Build history of the part. All positions in model axes, mm. A direction names the side the tool comes from. Round coordinates to 2 decimals unless told otherwise and drop trailing zeros. Write each loop counter-clockwise with the first axis right and the second up, starting at its lowest first coordinate (ties: lowest second). Pieces come first, ordered by that corner, then holes. Notation, with made-up numbers: (8.25, 21) - (32.25, 21) arc R25 ccw to (32.25, 49) - close; hole circle Ø8 at (72, 48). An arc over 180 degrees is marked (long way). Answer as a JSON object with one key per item and string values. Group by question number.
Item 1: Slice it at A-A, the plane x = 0. List the corners of the cut face in (y, z), then the cut area to 3 significant figures.
Item 2: Slice it at D-D, the plane y = -2.5. List the corners of the cut face in (x, z), then the cut area to 3 significant figures.
Item 3: Slice it at B-B, the plane y = 0. List the corners of the cut face in (x, z), then the cut area to 3 significant figures.
Item 4: Two-plate mould, pull along X, no slides. Class faces 6 (the flat face through (0, 2.524, 8)), 7 (the flat face through (-0.9, 2, -6)), 8 (the flat face through (0.9, 2, -6)): +X half, -X half, draft (parallel to the pull), parting line (faces both ways), or undercut.
Item 5: Probe line 1 (Y direction, x = 0, z = 5.75); line 2 (Z direction, x = -2.25, y = -0.5); line 3 (Z direction, x = -5.25, y = -5.5). List the from-to ranges inside material, lowest first. Write a range as from..to.
Item 6: Which spindle directions (+Z, -Z, +X, -X, +Y, -Y) get a long thin tool onto all of the face, cutting with end or side? Do faces 1 (the flat face through (-2, 0.9, -6)), 2 (the flat face through (0, 2.2, -6)), 3 (the flat face through (-0.9, -2, -6)), 4 (the flat face through (0, 0, 2)), 5 (the flat face through (0.9, -2, -6)). Say none if no direction does.
Item 7: Flat gauge pins, fed straight in: pin 1 (0.7 mm diameter, centred on y = -1.5, z = -4, fed in from -X); pin 2 (1 mm diameter, centred on x = -2, z = -6.5, fed in from +Y); pin 3 (6 mm diameter, centred on x = 3.5, z = 5, fed in from -Y). Where does each tip first touch, or does it go through?
Item 8: Slice it at C-C, the plane z = 5. List the corners of the cut face in (x, y), then the cut area to 3 significant figures.
from build123d import *

# Parameters (mm, degrees)
SKETCH_R     = 8
PAD_DEPTH    = 14
POCKET_DEPTH = 12
PAD001_DEPTH = 12


with BuildPart() as part:
    # Sketch → Pad (new body)
    with BuildSketch(Plane.XY):
        Circle(SKETCH_R)
    extrude(amount=PAD_DEPTH)

    # Sketch001 → Pocket (cut)
    with BuildSketch(Plane.XY.offset(14)):
        with BuildLine():
            Line((-1.8, 2.523886), (1.8, 2.523886))
            ThreePointArc((-1.8, 2.523886), (0, -3.1), (1.8, 2.523886))
        make_face()
    extrude(amount=-POCKET_DEPTH, mode=Mode.SUBTRACT)

    # Sketch002 → Pad001 (new body)
    with BuildSketch(Plane(origin=(0, 0, 0), x_dir=(1, 0, 0), z_dir=(0, 0, -1))):
        Polygon((-0.9, 2.2), (0.9, 2.2), (0.9, 0.9), (2.2, 0.9), (2.2, -0.9), (0.9, -0.9), (0.9, -2.2), (-0.9, -2.2), (-0.9, -0.9), (-2.2, -0.9), (-2.2, 0.9), (-0.9, 0.9), align=None)
    extrude(amount=PAD001_DEPTH)


solid = part.part
Geometry says:
{
 "1": {"outline": "(-8, 0) - (-2.2, 0) - (-2.2, -12) - (2.2, -12) - (2.2, 0) - (8, 0) - (8, 14) - (2.52, 14) - (2.52, 2) - (-3.1, 2) - (-3.1, 14) - (-8, 14) - close", "area": "209 mm^2"},
 "2": {"outline": "(-7.6, 0) - (7.6, 0) - (7.6, 14) - (1.83, 14) - (1.83, 2) - (-1.83, 2) - (-1.83, 14) - (-7.6, 14) - close", "area": "169 mm^2"},
 "3": {"outline": "(-8, 0) - (-2.2, 0) - (-2.2, -12) - (2.2, -12) - (2.2, 0) - (8, 0) - (8, 14) - (3.1, 14) - (3.1, 2) - (-3.1, 2) - (-3.1, 14) - (-8, 14) - close", "area": "202 mm^2"},
 "4": {"face 6": "undercut", "face 7": "-X half", "face 8": "+X half"},
 "5": {"line 1": "y = -8..-3.1, 2.52..8", "line 2": "z = 0..2", "line 3": "z = 0..14"},
 "6": {"face 1": "-Z, -X, +Y", "face 2": "-Z, +X, -X, +Y", "face 3": "-Z, -X, -Y", "face 4": "+Z", "face 5": "-Z, +X, -Y"},
 "7": {"pin 1": "stops at x = -0.9", "pin 2": "stops at y = 0.9", "pin 3": "stops at y = -7.98"},
 "8": {"outline": "circle Ø16 at (0, 0); hole (-1.8, 2.52) arc R3.1 ccw (long way) to (1.8, 2.52) - close", "area": "172 mm^2"}
}
